Could you check a few things on this model? Use its own coordinates, in mm. Round coordinates to 2 decimals unless told otherwise and drop trailing zeros. Loops run counter-clockwise (first coordinate to the right, second up) from the corner with the lowest first, then second, coordinate; pieces in that order, holes last. Notation, with made-up numbers: (-4.5, 78.25) -> (44.5, 78.25) arc R28 cw to (44.5, 113.25) -> close; hole circle Ø6 at (75, 29). An arc over 180 degrees is marked (long way). One line per item, written item: value.
from build123d import *

# Parameters (mm, degrees)
SKETCH020_W     = 14.1
SKETCH020_H     = 14.1
PAD014_DEPTH    = 2
SKETCH_W        = 14
SKETCH_H        = 2
PAD_DEPTH       = 1.9
SKETCH028_W     = 5
SKETCH028_H     = 0.8
POCKET004_DEPTH = 0.5


with BuildPart() as part:
    # Sketch020 → Pad014 (new body)
    with BuildSketch(Plane.XY):
        Polygon((39.7, 32.2), (39.7, -32.2), (-39.7, -32.2), (-39.7, 32.2), (-2.875, 32.2), (-2.875, 30.7), (-6.25, 30.7), (-6.25, 25.7), (6.25, 25.7), (6.25, 30.7), (2.875, 30.7), (2.875, 32.2), align=None)
        with Locations((-14.55, 16.1)):
            Rectangle(SKETCH020_W, SKETCH020_H, mode=Mode.SUBTRACT)
        with Locations((-14.55, 0)):
            Rectangle(SKETCH020_W, SKETCH020_H, mode=Mode.SUBTRACT)
        with Locations((-14.55, -16.1)):
            Rectangle(SKETCH020_W, SKETCH020_H, mode=Mode.SUBTRACT)
        with Locations((-30.65, -23.15)):
            Rectangle(SKETCH020_W, SKETCH020_H, mode=Mode.SUBTRACT)
        with Locations((-30.65, 23.15)):
            Rectangle(SKETCH020_W, SKETCH020_H, mode=Mode.SUBTRACT)
        with Locations((14.55, 16.1)):
            Rectangle(SKETCH020_W, SKETCH020_H, mode=Mode.SUBTRACT)
        with Locations((14.55, 0)):
            Rectangle(SKETCH020_W, SKETCH020_H, mode=Mode.SUBTRACT)
        with Locations((14.55, -16.1)):
            Rectangle(SKETCH020_W, SKETCH020_H, mode=Mode.SUBTRACT)
        with Locations((30.65, -23.15)):
            Rectangle(SKETCH020_W, SKETCH020_H, mode=Mode.SUBTRACT)
        with Locations((30.65, 23.15)):
            Rectangle(SKETCH020_W, SKETCH020_H, mode=Mode.SUBTRACT)
    extrude(amount=PAD014_DEPTH)

    # Sketch (on Face53 of Pad014) → Pad (join)
    with BuildSketch(Plane(origin=(0, 0, 0), x_dir=(1, 0, 0), z_dir=(0, 0, -1))):
        with Locations((0, -14)):
            Rectangle(SKETCH_W, SKETCH_H)
    extrude(amount=PAD_DEPTH)

    # Sketch028 (on Face4 of Pad) → Pocket004 (cut)
    with BuildSketch(Plane(origin=(0, 0, 0), x_dir=(1, 0, 0), z_dir=(0, 0, -1))):
        with Locations((-14.55, 7.45)):
            Rectangle(SKETCH028_W, SKETCH028_H)
        with Locations((-14.55, 8.65)):
            Rectangle(SKETCH028_W, SKETCH028_H)
        with Locations((-14.55, 23.55)):
            Rectangle(SKETCH028_W, SKETCH028_H)
        with Locations((-30.65, 30.6)):
            Rectangle(SKETCH028_W, SKETCH028_H)
        with Locations((-30.65, 15.7)):
            Rectangle(SKETCH028_W, SKETCH028_H)
        with Locations((-14.55, -7.45)):
            Rectangle(SKETCH028_W, SKETCH028_H)
        with Locations((-14.55, -8.65)):
            Rectangle(SKETCH028_W, SKETCH028_H)
        with Locations((-14.55, -23.55)):
            Rectangle(SKETCH028_W, SKETCH028_H)
        with Locations((-30.65, -30.6)):
            Rectangle(SKETCH028_W, SKETCH028_H)
        with Locations((-30.65, -15.7)):
            Rectangle(SKETCH028_W, SKETCH028_H)
    pocket004 = extrude(amount=-POCKET004_DEPTH, mode=Mode.SUBTRACT)

    # Mirrored: Pocket004 across Sketch028 V_Axis
    add(pocket004.mirror(Plane(origin=(0, 0, 0), x_dir=(0, 0, -1), z_dir=(1, 0, 0))), mode=Mode.SUBTRACT)


with BuildPart() as part_1:
    # Body005 placement: moved
    add(part.part.moved(Location((0, 0, -13.7))))


solid = part_1.part
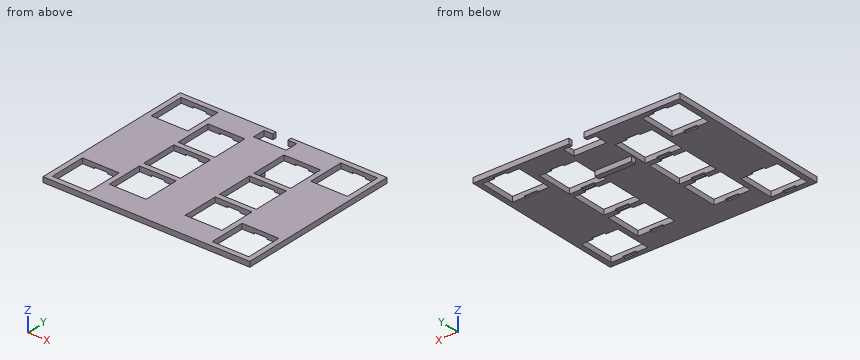
(1) I'm going to push a flat-ended pin straight in: pin 1 Ø5 at (x, y) = (-4, 9) entering from -Z. Where does the tip first touch, or does it pass through?
Recorded:
pin 1: z = -13.7
(2) If we section it at A-A, the plane x = 34: Please give me the cut outline in (y, z), then the cut area to 3 significant figures.
Recorded:
outline: (-32.2, -13.7) -> (-30.2, -13.7) -> (-30.2, -11.7) -> (-32.2, -11.7) -> close; (-16.1, -13.7) -> (16.1, -13.7) -> (16.1, -11.7) -> (-16.1, -11.7) -> close; (30.2, -13.7) -> (32.2, -13.7) -> (32.2, -11.7) -> (30.2, -11.7) -> close
area: 72.4 mm²
(3) If I drill on L1, parallel to X at y = -7, z = -11.85; L2, parallel to Y at x = 18.5, z = -12.2; L3, parallel to Y at x = -14, z = -13.35, over which ranges is the centre line in solid material (lowest first)?
Recorded:
L1: -39.7 to -21.6, -7.5 to 7.5, 21.6 to 39.7
L2: -32.2 to -23.15, -9.05 to -7.05, 7.05 to 9.05, 23.15 to 32.2
L3: -32.2 to -23.95, -8.25 to -7.85, 7.85 to 8.25, 23.95 to 32.2
(4) If we section it at D-D, the plane y = 3.5: Please give me the cut outline in (x, z), then the cut area to 3 significant figures.
Recorded:
outline: (-39.7, -13.7) -> (-21.6, -13.7) -> (-21.6, -11.7) -> (-39.7, -11.7) -> close; (-7.5, -13.7) -> (7.5, -13.7) -> (7.5, -11.7) -> (-7.5, -11.7) -> close; (21.6, -13.7) -> (39.7, -13.7) -> (39.7, -11.7) -> (21.6, -11.7) -> close
area: 102 mm²
(5) If we section it at B-B, the plane y = 21: Please give me the cut outline in (x, z), then the cut area to 3 significant figures.
Recorded:
outline: (-39.7, -13.7) -> (-37.7, -13.7) -> (-37.7, -11.7) -> (-39.7, -11.7) -> close; (-23.6, -13.7) -> (-21.6, -13.7) -> (-21.6, -11.7) -> (-23.6, -11.7) -> close; (-7.5, -13.7) -> (7.5, -13.7) -> (7.5, -11.7) -> (-7.5, -11.7) -> close; (21.6, -13.7) -> (23.6, -13.7) -> (23.6, -11.7) -> (21.6, -11.7) -> close; (37.7, -13.7) -> (39.7, -13.7) -> (39.7, -11.7) -> (37.7, -11.7) -> close
area: 46.0 mm²
(6) If we section it at C-C, the plane x = 9: Please give me the cut outline in (y, z).
Recorded:
outline: (-32.2, -13.7) -> (-23.15, -13.7) -> (-23.15, -11.7) -> (-32.2, -11.7) -> close; (-9.05, -13.7) -> (-7.05, -13.7) -> (-7.05, -11.7) -> (-9.05, -11.7) -> close; (7.05, -13.7) -> (9.05, -13.7) -> (9.05, -11.7) -> (7.05, -11.7) -> close; (23.15, -13.7) -> (32.2, -13.7) -> (32.2, -11.7) -> (23.15, -11.7) -> close
